Source: CAD feature listing. Evaluate the final solid. Frame: model axes, mm. A direction names the side the tool comes from. Give positions to 0.01 mm unless a question says otherwise; leave off trailing zeros. Loops run counter-clockwise (first coordinate to the right, second up) from the corner with the lowest first, then second, coordinate; pieces in that order, holes last. Notation, with made-up numbers: (-25.5, 70) - (30.5, 70) arc R16 ccw to (30.5, 89) - close; hole circle Ø8 at (58, 23.25). An arc over 180 degrees is marked (long way). Put each result on its own line as item: value.
```python
from build123d import *

# Parameters (mm, degrees)
SKETCH_W     = 7.5
SKETCH_H     = 7.5
SKETCH_W_2   = 6.05
SKETCH_H_2   = 6.05
PAD_DEPTH    = 3.05
SKETCH001_W  = 7.5
SKETCH001_H  = 7.5
PAD001_DEPTH = 0.95
SKETCH002_W  = 7
SKETCH002_H  = 2
PAD002_DEPTH = 6
SKETCH004_W  = 7
SKETCH004_H  = 2
PAD003_DEPTH = 6
SKETCH005_R  = 1.7
HOLE_DEPTH   = 25
SKETCH006_R  = 2
POCKET_DEPTH = 1


with BuildPart() as part:
    # Sketch → Pad (new body)
    with BuildSketch(Plane.XY):
        Rectangle(SKETCH_W, SKETCH_H)
        Rectangle(SKETCH_W_2, SKETCH_H_2, mode=Mode.SUBTRACT)
    extrude(amount=PAD_DEPTH)

    # Sketch001 (on Face10 of Pad) → Pad001 (join)
    with BuildSketch(Plane.XY.offset(3.05)):
        Rectangle(SKETCH001_W, SKETCH001_H)
    extrude(amount=PAD001_DEPTH)

    # Sketch002 (on Face10 of Pad001) → Pad002 (join)
    with BuildSketch(Plane.XZ.offset(3.75)):
        with Locations((-0.25, 1)):
            Rectangle(SKETCH002_W, SKETCH002_H)
    extrude(amount=PAD002_DEPTH)

    # Sketch004 (on Face2 of Pad002) → Pad003 (join)
    with BuildSketch(Plane.YZ.offset(3.75)):
        with Locations((0.25, 1)):
            Rectangle(SKETCH004_W, SKETCH004_H)
    extrude(amount=PAD003_DEPTH)

    # Sketch005 (on Face11 of Pad003) → Hole (cut)
    with BuildSketch(Plane(origin=(0, 0, 0), x_dir=(1, 0, 0), z_dir=(0, 0, -1))):
        with Locations((6.75, -0.25)):
            Circle(SKETCH005_R)
        with Locations((-0.25, 6.75)):
            Circle(SKETCH005_R)
    extrude(amount=-HOLE_DEPTH, mode=Mode.SUBTRACT)

    # Sketch006 (on Face3 of Hole) → Pocket (cut)
    with BuildSketch(Plane.XY.offset(4)):
        Circle(SKETCH006_R)
    extrude(amount=-POCKET_DEPTH, mode=Mode.SUBTRACT)


solid = part.part
```
1) Material intervals for line 1 along X through (y, z) = (0.25, 1.15) (3 decimals); line 2 along Y through (x, z) = (0.25, 1.05) (3 decimals); line 3 along Y through (x, z) = (2, 2.2) (3 decimals), sorted ascending. Write a range as [from, to].
Check result:
line 1: [-3.75, -3.025], [3.025, 5.05], [8.45, 9.75]
line 2: [-9.75, -8.375], [-5.125, -3.025], [3.025, 3.75]
line 3: [-3.75, -3.025], [3.025, 3.75]
2) Section query B-B, the plane x = 5.5. Output: boundary loops of the cut face in (y, z), plus the area to 3 significant figures.
Check result:
outline: (-3.25, 0) - (-0.9, 0) - (-0.9, 2) - (-3.25, 2) - close; (1.4, 0) - (3.75, 0) - (3.75, 2) - (1.4, 2) - close
area: 9.39 mm²
3) Pin query (flat end, axial travel): P1, Ø0.6, axis at x = 6, z = 1, coming from the -Y side; P2, Ø5, axis at x = 0, y = 0, coming from the -Z side; P3, Ø4, axis at x = 6.75, y = 0.25, coming from the +Z side. Return the tip coordinate at first contact, or that it passes through.
Check result:
P1: y = -3.25
P2: z = 3.05
P3: z = 2
4) Section query C-C, the plane y = 0.25. Output: boundary loops of the cut face in (x, z) (3 decimals).
Check result:
outline: (-3.75, 0) - (-3.025, 0) - (-3.025, 3.05) - (-1.984, 3.05) - (-1.984, 4) - (-3.75, 4) - close; (1.984, 3.05) - (3.025, 3.05) - (3.025, 0) - (5.05, 0) - (5.05, 2) - (3.75, 2) - (3.75, 4) - (1.984, 4) - close; (8.45, 0) - (9.75, 0) - (9.75, 2) - (8.45, 2) - close
5) Section query D-D, the plane z = 1.75. Output: boundary loops of the cut face in (x, y) (3 decimals).
Check result:
outline: (-3.75, -9.75) - (3.25, -9.75) - (3.25, -3.75) - (3.75, -3.75) - (3.75, -3.25) - (9.75, -3.25) - (9.75, 3.75) - (-3.75, 3.75) - close; hole (-3.025, -3.025) - (3.025, -3.025) - (3.025, 3.025) - (-3.025, 3.025) - close; hole circle Ø3.4 at (-0.25, -6.75); hole circle Ø3.4 at (6.75, 0.25)
6) Mould query, pull axis X, two halves, no side actions, for faces 4 (the flat face through (3.025, 0, 2)), 5 (the flat face through (9.75, 0, 1)), 6 (the flat face through (9, 0, 2)). Classes: pulls with the +X half, pulls with the -X half, needs draft (parallel to the pull), parting line crosses it, or undercut.
Check result:
face 4: undercut
face 5: pulls with the +X half
face 6: needs draft
7) Section query A-A, the plane y = -6.75. Output: boundary loops of the cut face in (x, z), plus the area to 3 significant figures.
Check result:
outline: (-3.75, 0) - (-1.95, 0) - (-1.95, 2) - (-3.75, 2) - close; (1.45, 0) - (3.25, 0) - (3.25, 2) - (1.45, 2) - close
area: 7.20 mm²
8) Access query for faces 1 (the flat face through (0, -3.025, 2)), 2 (the flat face through (7, -3.25, 1)), 3 (the flat face through (-2, -6, 2)). Directions: +Z, -Z, +X, -X, +Y, -Y. A direction counts if a zero-diameter tool reaches every point of the face in a straight line with its end or side. Return the directions, or none.
Check result:
face 1: -Z
face 2: +Z, -Z, +X, -Y
face 3: +Z, +X, -X, -Y
